```python
from build123d import *

# Parameters (mm, degrees)
F1_DEPTH = 29
F4_DEPTH = 2
F3_R     = 2.5
F5_DEPTH = 2


with BuildPart() as f1:
    # F0 (on Top) → F1 (new body)
    with BuildSketch(Plane.XY):
        with BuildLine():
            ThreePointArc((-15.034174097, 47.3746718097), (-14.5746321535, 50.8652394172), (-16.7178909544, 53.6583886671))
            Line((-16.7178909544, 53.6583886671), (-36.4632701607, 65.0583886671))
            ThreePointArc((-36.4632701607, 65.0583886671), (-37.6773806328, 65.2182293432), (-38.6489108067, 64.4727480211))
            Line((-38.6489108067, 64.4727480211), (-59.9489108067, 27.5800658199))
            Line((-59.9489108067, 27.5800658199), (-61.2528943298, 25.3215001057))
            ThreePointArc((-61.2528943298, 25.3215001057), (-61.8042473465, 21.739302036), (-59.7906494926, 18.7257398843))
            Line((-59.7906494926, 18.7257398843), (-47.1451993997, 9.8713004052))
            ThreePointArc((-47.1451993997, 9.8713004052), (-44.962234305, 8.7947811535), (-42.5565879089, 8.4245167595))
            Line((-42.5565879089, 8.4245167595), (-32.4906988756, 8.4245167595))
            ThreePointArc((-32.4906988756, 8.4245167595), (-28.9976482356, 9.8470040444), (-27.492125644, 13.3050778688))
            Line((-27.492125644, 13.3050778688), (-27.2173277766, 24.8054966721))
            ThreePointArc((-27.2173277766, 24.8054966721), (-26.9956322368, 26.2841998916), (-26.4151923214, 27.6621700032))
            Line((-26.4151923214, 27.6621700032), (-15.034174097, 47.3746718097))
        make_face()
        with BuildLine():
            Line((-58.5632701607, 26.7800658199), (-40.3767366812, 16.2800658199))
            ThreePointArc((-40.3767366812, 16.2800658199), (-39.162626209, 16.1202251439), (-38.1910960352, 16.8657064659))
            Line((-38.1910960352, 16.8657064659), (-17.6910960352, 52.3727480211))
            Line((-17.6910960352, 52.3727480211), (-17.5178909544, 52.2727480211))
            ThreePointArc((-17.5178909544, 52.2727480211), (-16.1201134755, 50.451128945), (-16.419814743, 48.1746718097))
            Line((-16.419814743, 48.1746718097), (-28.1671840961, 27.8276312349))
            ThreePointArc((-28.1671840961, 27.8276312349), (-28.9411039834, 25.9903377528), (-29.2366980364, 24.01873346))
            Line((-29.2366980364, 24.01873346), (-29.4437657435, 15.3528534251))
            ThreePointArc((-29.4437657435, 15.3528534251), (-30.3470792985, 13.2780091304), (-32.4429096825, 12.4245167595))
            Line((-32.4429096825, 12.4245167595), (-41.9259903312, 12.4245167595))
            ThreePointArc((-41.9259903312, 12.4245167595), (-43.7302251282, 12.702215055), (-45.3674489493, 13.5096044937))
            Line((-45.3674489493, 13.5096044937), (-57.9685892112, 22.3330178952))
            ThreePointArc((-57.9685892112, 22.3330178952), (-59.1767479235, 24.1411551862), (-58.8459361135, 26.290474028))
            Line((-58.8459361135, 26.290474028), (-58.5632701607, 26.7800658199))
        make_face(mode=Mode.SUBTRACT)
        Polygon((-37.2632701607, 63.6727480211), (-19.0767366812, 53.1727480211), (-39.5767366812, 17.6657064659), (-57.7632701607, 28.1657064659), align=None, mode=Mode.SUBTRACT)
    extrude(amount=F1_DEPTH)

    # F2 (on face) → F4 (cut)
    with BuildSketch(Plane(origin=(-56.9042019241, 32.8536562989, 0), x_dir=(-0.5, -0.8660254038, 0), z_dir=(-0.8660254038, 0.5, 0))):
        with BuildLine():
            ThreePointArc((-36.0013197979, 29), (-36.0082664269, 28.7500428927), (-36.0105822347, 28.5))
            ThreePointArc((-36.0105822347, 28.5), (-22.5105822347, 15), (-9.0105822347, 28.5))
            ThreePointArc((-9.0105822347, 28.5), (-9.0128980425, 28.7500428927), (-9.0198446715, 29))
            Line((-9.0198446715, 29), (-36.0013197979, 29))
        make_face()
        with BuildLine():
            ThreePointArc((-9.0198446715, 29), (-9.0128980425, 28.7500428927), (-9.0105822347, 28.5))
            Line((-9.0105822347, 28.5), (-9.0105822347, 29))
            Line((-9.0105822347, 29), (-9.0198446715, 29))
        make_face()
        with BuildLine():
            ThreePointArc((-14.496704046, 0), (-23.5105822347, 6.5), (-32.5244604233, 0))
            Line((-32.5244604233, 0), (-14.496704046, 0))
        make_face()
    extrude(amount=-F4_DEPTH, mode=Mode.SUBTRACT)

    # F3 (on face) → F5 (cut)
    with BuildSketch(Plane(origin=(19.0552911173, 33.0047323683, 0), x_dir=(-0.8660254038, 0.5, 0), z_dir=(0.5, 0.8660254038, 0))):
        with BuildLine():
            Line((45.6529565405, 0), (56.5616686551, 0))
            ThreePointArc((56.5616686551, 0), (51.1073125978, 3.5), (45.6529565405, 0))
        make_face()
        with Locations((57.1073125978, 5.5)):
            Circle(F3_R)
    extrude(amount=-F5_DEPTH, mode=Mode.SUBTRACT)


solid = f1.part
```
Geometry check sheet. Reference: the model listing, model coordinates, mm. A direction names the side the tool comes from. Give positions to 0.01 mm unless a question says otherwise; leave off trailing zeros. Write each loop counter-clockwise with the first axis right and the second up, starting at its lowest first coordinate (ties: lowest second). Pieces come first, ordered by that corner, then holes.
1) Section check D-D, the plane y = 20. Record the boundary of the cut face in (x, z), and give its area (3 significant figures).
2) Gauge pin test, flat ends, axial feed: pin 1 (5 mm diameter, centred on x = -47.5, z = 25, fed in from -Y); pin 2 (4 mm diameter, centred on y = 47, z = 19.5, fed in from +X); pin 3 (1 mm diameter, centred on x = -45.5, y = 48.5, fed in from +Z). Record the tip position at first contact, or that the pin passes through.
3) Material ranges on L1, parallel to Y at x = -33.5, z = 8; L2, parallel to Y at x = -33, z = 10.5; L3, parallel to X at y = 30.5, z = 18.5, recorded low to high.
4) Release check for a two-part mould opening along Y. For faces 1 (the cylindrical face through (-44.5, 52.7, 6.5)), 2 (the cylindrical face through (-14.562, 50.816, 14.297)), 3 (the flat face through (-53.556, 14.361, 14.297)), 4 (the flat face through (-26.452, 59.279, 14.297)) record: pulls with the +Y half, pulls with the -Y half, needs draft (parallel to the pull), parting line crosses it, or undercut.
5) Section check C-C, the plane y = 31.5. Record the boundary of the cut face in (x, z), and give its area (3 significant figures).
6) Section check B-B, the plane x = -54.5. Record the boundary of the cut face in (y, z), and give its area (3 significant figures).
7) Section check A-A, the plane z = 11.25. State how many separate pieces and enclosed holes the cut face has, and give its area (3 significant figures).
8) Access from +Z, -Z, +X, -X, +Y, -Y to the whole of each face (thin tool, end or side, straight path). Record for faces 5 (the cylindrical face through (-39.18, 16.116, 14.297)), 6 (the flat face through (-38, 8.425, 14)).
Computed:
1. outline: (-61.05, 0) - (-54.64, 0) - (-54.64, 29) - (-61.05, 29) - close; (-46.82, 0) - (-43.62, 0) - (-43.62, 29) - (-46.82, 29) - close; (-38.23, 0) - (-36.38, 0) - (-36.38, 29) - (-38.23, 29) - close; (-29.33, 0) - (-27.33, 0) - (-27.33, 29) - (-29.33, 29) - close
1. area: 390 mm2
2. pin 1: stops at y = 8.81
2. pin 2: stops at x = -14.47
2. pin 3: stops at z = 15.45
3. L1: y = 8.42 to 12.42, 24.99 to 28.19, 61.5 to 63.35
3. L2: y = 8.42 to 12.42, 25.86 to 29.06, 61.21 to 63.06
3. L3: x = -58.26 to -56.42, -32.17 to -30.32, -26.62 to -24.78
4. face 1: undercut
4. face 2: parting line crosses it
4. face 3: pulls with the -Y half
4. face 4: pulls with the +Y half
5. outline: (-57.69, 0) - (-55.84, 0) - (-55.84, 29) - (-57.69, 29) - close; (-31.59, 0) - (-29.74, 0) - (-29.74, 29) - (-31.59, 29) - close; (-26.05, 0) - (-24.2, 0) - (-24.2, 29) - (-26.05, 29) - close
5. area: 161 mm2
6. outline: (15.02, 0) - (19.9, 0) - (19.9, 29) - (15.02, 29) - close; (24.43, 0) - (26.28, 0) - (26.28, 29) - (24.43, 29) - close; (33.82, 0) - (37.02, 0) - (37.02, 29) - (33.82, 29) - close
6. area: 288 mm2
7. separate pieces: 1
7. enclosed holes: 2
7. area: 439 mm2
8. face 5: +Z, -Z
8. face 6: +Z, -Z, +X, -X, -Y
